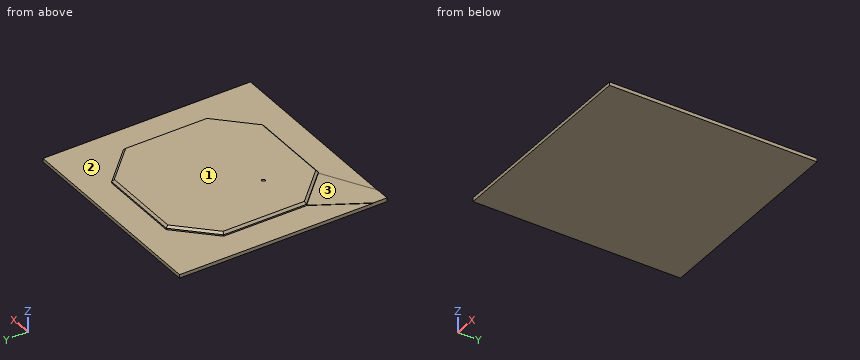
Autodesk Inventor part; units mm, degrees
ref_plane "YZ Plane" through (0, 0, 0) normal (1, 0, 0) x (0, 1, 0)
ref_plane "XZ Plane" through (0, 0, 0) normal (0, 1, 0) x (-1, 0, 0)
ref_plane "XY Plane" through (0, 0, 0) normal (0, 0, 1) x (1, 0, 0)
sketch "Sketch1" plane through (0, 0, 0) normal (0, 0, 1) x (1, 0, 0)
  line L0 (0, 24) -> (0, -18)
  line L1 (-18, 0) -> (24, 0)
  line L2 (-15, 15) -> (15, 15)
  line L3 (15, 15) -> (15, -15)
  line L4 (15, -15) -> (-15, -15)
  line L5 (-15, -15) -> (-15, 15)
  dimension "d0" = 30
extrude "Extrusion1" add sketch "Sketch1" along normal blind 0.5
sketch "Sketch2" plane through (0, 0, 0.5) normal (0, 0, 1) x (1, 0, 0)
  line L0 (0, 24) -> (0, -18)
  line L1 (-18, 0) -> (24, 0)
  line L2 (-11, 11) -> (11, 11)
  line L3 (11, 11) -> (11, -11)
  line L4 (11, -11) -> (-11, -11)
  line L5 (-11, -11) -> (-11, 11)
  dimension "d3" = 22
extrude "Extrusion2" add sketch "Sketch2" along normal blind 0.5
chamfer "Chamfer1" distance 5 angle 45 4 edges at (-11, -11, 0.75) (11, -11, 0.75) (11, 11, 0.75) (-11, 11, 0.75)
chamfer "Chamfer2" distance 0.3 angle 45 8 edges at (-11, 0, 1) (-8.5, -8.5, 1) (0, -11, 1) (8.5, -8.5, 1) (11, 0, 1) (8.5, 8.5, 1) (0, 11, 1) (-8.5, 8.5, 1)
sketch "Sketch3" plane through (0, 0, 0.5) normal (0, 0, 1) x (1, 0, 0)
  line L0 (-11, -6) -> (-6, -11)
  line L1 (-15, -15) -> (-15, 15)
  line L2 (15, -15) -> (-15, -15)
  line L3 (-11, -6) -> (-15, -13)
  line L4 (-6, -11) -> (-13, -15)
  dimension "d12" = 2
  dimension "d13" = 2
extrude "Extrusion3" add sketch "Sketch3" along normal blind 0.05
sketch "Sketch4" plane through (0, 0, 1) normal (0, 0, 1) x (1, 0, 0)
  circle A0 centre (-4.2146, -4.2224) radius 0.25
  dimension "d16" = 0.5
extrude "Extrusion4" cut sketch "Sketch4" against normal blind 0.1
fillet "Fillet1" radius 0.1 1 edges at (-4.4646, -4.2224, 0.9)
equation "\"d13\" = d12"
properties part number "config - chip 15 x15"
Design review of the part built by this model. Coordinates are the model's own, in mm. Face numbers are marked on the shaded views. A direction names the side the tool comes from. Round coordinates to 2 decimals unless told otherwise and drop trailing zeros. Order: outer loops, then holes, each group sorted by start corner. A loop starts at its lowest first (then second) coordinate and runs counter-clockwise, first axis right, second up. Notation, with made-up numbers: (25, 61.5) - (42, 61.5) arc R27 cw to (42, 86.5) - close; hole circle Ø2 at (56.5, 41.25). An arc over 180 degrees is marked (long way). Return JSON: item names as keys, results as strings.
Q1. Wall thickness on L1, parallel to Z at x = -12.5, y = 10.5; L2, parallel to Y at x = -2, z = 0.6; L3, parallel to Z at x = -11, y = -12.75: over which ranges is each line inside the solid? List them lowest first. Write a range as [from, to].
Computed values:
{"L1": "z = [0, 0.5]", "L2": "y = [-11, 11]", "L3": "z = [0, 0.55]"}
Q2. Consider section A-A on x = -0.25. Write out the cut boundary in (y, z).
Computed values:
{"outline": "(-15, 0) - (15, 0) - (15, 0.5) - (11, 0.5) - (11, 0.7) - (10.7, 1) - (-10.7, 1) - (-11, 0.7) - (-11, 0.5) - (-15, 0.5) - close"}
Q3. Consider section D-D on y = -6.5. Write out the cut boundary in (x, z), plus the area to 3 significant figures.
Computed values:
{"outline": "(-15, 0) - (15, 0) - (15, 0.5) - (10.5, 0.5) - (10.5, 0.7) - (10.08, 1) - (-10.08, 1) - (-10.5, 0.7) - (-10.5, 0.55) - (-11.29, 0.55) - (-11.29, 0.5) - (-15, 0.5) - close", "area": "25.4 mm2"}
Q4. Machinability: for the marked faces 1, 2 and 3, which of the approach directions +Z, -Z, +X, -X, +Y, -Y give a long, thin tool a straight path to every point of the face, cutting with its end or side? Answer none if there is none.
Computed values:
{"face 1": "+Z, +X, -X, +Y, -Y", "face 2": "+Z", "face 3": "+Z, -X, -Y"}
Q5. Consider section C-C on x = -7.5. Write out the cut boundary in (y, z).
Computed values:
{"outline": "(-15, 0) - (15, 0) - (15, 0.5) - (9.5, 0.5) - (9.5, 0.7) - (9.08, 1) - (-9.08, 1) - (-9.5, 0.7) - (-9.5, 0.55) - (-11.86, 0.55) - (-11.86, 0.5) - (-15, 0.5) - close"}
Q6. For pin 1 Ø3 at (x, y) = (-4.5, 11) entering from -Z; pin 2 Ø1.5 at (x, y) = (0, -12) entering from +Z; pin 3 Ø4.5 at (x, y) = (-11.5, -9.5) entering from +Z, all flat-tipped, find the tip position at first contact; note any pin that passes through.
Computed values:
{"pin 1": "stops at z = 0", "pin 2": "stops at z = 0.5", "pin 3": "stops at z = 0.55"}
